Geometry: final body of the model. Coordinates: model frame, mm. Face numbers are marked on the shaded views. Round coordinates to 2 decimals unless told otherwise and drop trailing zeros. Loops run counter-clockwise (first coordinate to the right, second up) from the corner with the lowest first, then second, coordinate; pieces in that order, holes last. Notation, with made-up numbers: M 75,-22 L 86,-22 A17 cw 86,11 Z; hole C -38,-25 d10. An arc over 180 degrees is marked long. Return JSON: item names as keys, results as strings.
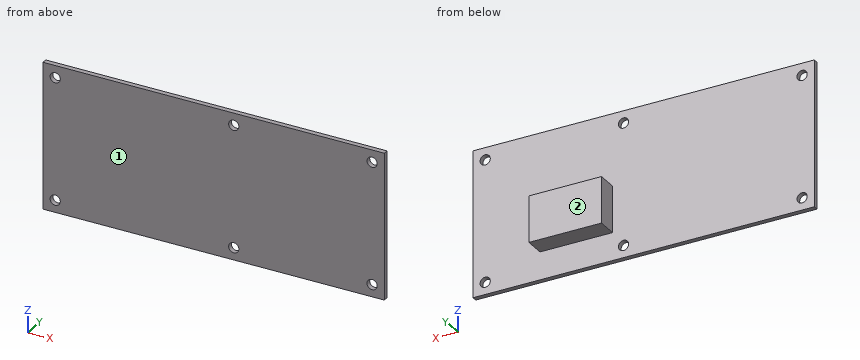
from build123d import *

# Parameters (mm, degrees)
SKETCH1_W           = 140
SKETCH1_H           = 60
SKETCH1_R           = 2.0955
BOSS_EXTRUDE1_DEPTH = 2
SKETCH2_W           = 29.777089478
SKETCH2_H           = 19.000212295
BOSS_EXTRUDE2_DEPTH = 8.174


with BuildPart() as part:
    # Sketch1 → Boss-Extrude1 (new body)
    with BuildSketch(Plane(origin=(0, 0, 0), x_dir=(1, 0, 0), z_dir=(0, 1, 0))):
        with Locations((-8.25, 0)):
            Rectangle(SKETCH1_W, SKETCH1_H)
        with Locations(Location((-73.25, 25, 0), (0, 0, 270))):
            Circle(SKETCH1_R, mode=Mode.SUBTRACT)
        with Locations(Location((-73.25, -25, 0), (0, 0, 270))):
            Circle(SKETCH1_R, mode=Mode.SUBTRACT)
        with Locations(Location((0, 25, 0), (0, 0, 270))):
            Circle(SKETCH1_R, mode=Mode.SUBTRACT)
        with Locations(Location((0, -25, 0), (0, 0, 270))):
            Circle(SKETCH1_R, mode=Mode.SUBTRACT)
        with Locations(Location((56.75, 25, 0), (0, 0, 270))):
            Circle(SKETCH1_R, mode=Mode.SUBTRACT)
        with Locations(Location((56.75, -25, 0), (0, 0, 270))):
            Circle(SKETCH1_R, mode=Mode.SUBTRACT)
    extrude(amount=BOSS_EXTRUDE1_DEPTH)

    # Sketch2 → Boss-Extrude2 (add)
    with BuildSketch(Plane(origin=(0, 2, 0), x_dir=(1, 0, 0), z_dir=(0, 1, 0))):
        with Locations((19.386769675, 9.085304713)):
            Rectangle(SKETCH2_W, SKETCH2_H)
    extrude(amount=BOSS_EXTRUDE2_DEPTH)


solid = part.part
Q1. Pin query (flat end, axial travel): pin 1 (1.5 mm diameter, centred on x = 0, z = -21, fed in from +Y); pin 2 (2.5 mm diameter, centred on y = 7, z = -11.5, fed in from -X); pin 3 (3.5 mm diameter, centred on x = 0, z = -25, fed in from +Y); pin 4 (5 mm diameter, centred on x = 9, y = 6.5, fed in from -Z). Return the tip coordinate at first contact, or that it passes through.
Determined:
{"pin 1": "stops at y = 2", "pin 2": "stops at x = 4.5", "pin 3": "passes through", "pin 4": "stops at z = -18.59"}
Q2. Section query A-A (z = 25). Output: boundary loops of the cut face in (x, y).
Determined:
{"outline": "M -78.25,0 L -75.35,0 L -75.35,2 L -78.25,2 Z; M -71.15,0 L -2.1,0 L -2.1,2 L -71.15,2 Z; M 2.1,0 L 54.65,0 L 54.65,2 L 2.1,2 Z; M 58.85,0 L 61.75,0 L 61.75,2 L 58.85,2 Z"}
Q3. Material intervals for L1, parallel to X at y = 1.15, z = 25; L2, parallel to Y at x = 4, z = 0; L3, parallel to X at y = 2.25, z = -3, sorted ascending.
Determined:
{"L1": "x = -78.25 to -75.35, -71.15 to -2.1, 2.1 to 54.65, 58.85 to 61.75", "L2": "y = 0 to 2", "L3": "x = 4.5 to 34.28"}
Q4. Section query D-D (y = 7). Output: boundary loops of the cut face in (x, z), plus the area to 3 significant figures.
Determined:
{"outline": "M 4.5,-18.59 L 34.28,-18.59 L 34.28,0.41 L 4.5,0.41 Z", "area": "566 mm^2"}
Q5. Pull-direction query (Y, two-part tool) for the marked faces 1 and 2; classes: pulls with the +Y half, pulls with the -Y half, needs draft (parallel to the pull), parting line crosses it, or undercut.
Determined:
{"face 1": "pulls with the -Y half", "face 2": "pulls with the +Y half"}
Q6. Section query C-C (z = -2). Output: boundary loops of the cut face in (x, y).
Determined:
{"outline": "M -78.25,0 L 61.75,0 L 61.75,2 L 34.28,2 L 34.28,10.17 L 4.5,10.17 L 4.5,2 L -78.25,2 Z"}
Q7. Section query B-B (x = 0). Output: boundary loops of the cut face in (y, z), plus the area to 3 significant figures.
Determined:
{"outline": "M 0,-30 L 2,-30 L 2,-27.1 L 0,-27.1 Z; M 0,-22.9 L 2,-22.9 L 2,22.9 L 0,22.9 Z; M 0,27.1 L 2,27.1 L 2,30 L 0,30 Z", "area": "103 mm^2"}
